Design review of the part built by this model. Coordinates are the model's own, in mm. Give positions to 0.01 mm unless a question says otherwise; leave off trailing zeros. Write each loop counter-clockwise with the first axis right and the second up, starting at its lowest first coordinate (ties: lowest second). Pieces come first, ordered by that corner, then holes. Notation, with made-up numbers: M 67,-39 L 78,-39 A21 ccw 78,-35 Z; hole C 40.5,-27 d3. An arc over 180 degrees is marked long. Use a Markdown table: item, result. Add a question column.
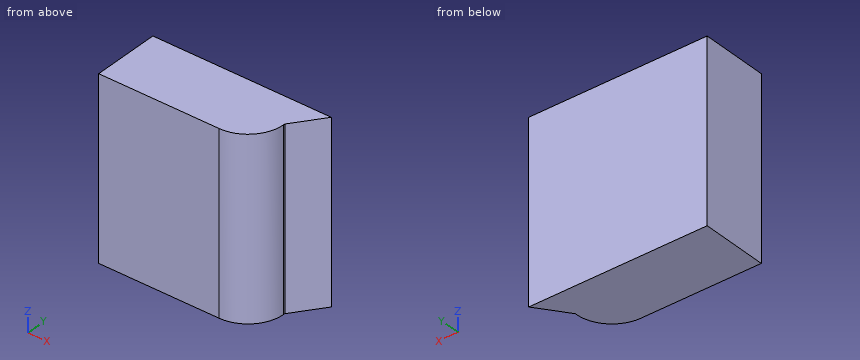
```python
from build123d import *

# Parameters (mm, degrees)
BOSS_EXTRUDE1_DEPTH = 40
FILLET1_R           = 8


with BuildPart() as part:
    # Sketch1 → Boss-Extrude1 (new body)
    with BuildSketch(Plane.XY):
        Polygon((-13.768148554, -75.866074504), (26.231851446, -75.866074504), (21.231851446, -82.575243148), (21.231851446, -90.866074504), (-13.768148554, -90.866074504), align=None)
    extrude(amount=BOSS_EXTRUDE1_DEPTH)

    # Fillet1
    fillet1_edges = [part.edges().sort_by_distance(p)[0] for p in [
        (21.231851446, -90.866074504, 20),
    ]]
    fillet(fillet1_edges, radius=FILLET1_R)


solid = part.part
```
(1) Add section A-A on z = 27. Give the boundary of the cut face in (x, y).
(2) For pin 1 (5 mm diameter, centred on y = -80, z = 26.5, fed in from +X); pin 2 (2 mm diameter, centred on y = -87.5, z = 13.5, fed in from +X); pin 3 (5 mm diameter, centred on y = -82, z = 21, fed in from +X), all flat-tipped, find the tip position at first contact; note any pin that passes through.
(3) Wall thickness on L1, parallel to Y at x = 13.5, z = 32; L2, parallel to X at y = -83, z = 19; L3, parallel to X at y = -77, z = 25.5: over which ranges is each line inside the solid? List them lowest first.
(4) Add section C-C on x = 23. Give the boundary of the cut face in (y, z), then the cut area to 3 significant figures.
(5) Add section B-B on y = -79.5. Give the boundary of the cut face in (x, z), then the cut area to 3 significant figures.
From the geometry:
| question | item | result |
|---|---|---|
| 1 | outline | M -13.77,-90.87 L 13.23,-90.87 A8 ccw 21.23,-82.87 L 21.23,-82.58 L 26.23,-75.87 L -13.77,-75.87 Z |
| 2 | pin 1 | stops at x = 25.01 |
| 2 | pin 2 | stops at x = 20.36 |
| 2 | pin 3 | stops at x = 23.52 |
| 3 | L1 | y = -90.86 to -75.87 |
| 3 | L2 | x = -13.77 to 21.23 |
| 3 | L3 | x = -13.77 to 25.39 |
| 4 | outline | M -80.2,0 L -75.87,0 L -75.87,40 L -80.2,40 Z |
| 4 | area | 173 mm^2 |
| 5 | outline | M -13.77,0 L 23.52,0 L 23.52,40 L -13.77,40 Z |
| 5 | area | 1,490 mm^2 |
